The listing builds one solid part. Answer for the finished solid, in the listing's coordinates (mm). A direction names the side the tool comes from. Coordinates: 2 decimals unless noted, no trailing zeros. Write each loop counter-clockwise with the first axis right and the second up, starting at its lowest first coordinate (ties: lowest second). Pieces come first, ordered by that corner, then holes.
from build123d import *

# Parameters (mm, degrees)
BOSS_EXTRUDE1_DEPTH = 4.365625
SKETCH2_OUTSIDE_W   = 44.614
SKETCH2_OUTSIDE_H   = 45.964
SKETCH2_OUTSIDE_R   = 4.365625
CUT_EXTRUDE1_DEPTH  = 8.9705043
CUT_EXTRUDE1_DRAFT  = -60
SKETCH4_R           = 2.0828
CUT_EXTRUDE3_DEPTH  = 4.365625
SKETCH9_W           = 1.767564538
SKETCH9_H           = 1.190625


# Read off the part's stored shape, not the designer's step: Cut-Extrude4, Cut-Extrude5
with BuildPart() as part:
    # Sketch1 → Boss-Extrude1 (new body)
    with BuildSketch(Plane(origin=(0, 0, 0), x_dir=(1, 0, 0), z_dir=(0, 1, 0))):
        Polygon((0, 5.040989538), (-4.365625, 2.520494769), (-4.365625, -2.520494769), (0, -5.040989538), (4.365625, -2.520494769), (4.365625, 2.520494769), align=None)
    extrude(amount=BOSS_EXTRUDE1_DEPTH)


with BuildPart() as cut_extrude1_tool:
    # Sketch2 outside → Cut-Extrude1 (with draft: the straight prism first)
    with BuildSketch(Plane(origin=(0, 4.365625, 0), x_dir=(1, 0, 0), z_dir=(0, 1, 0))):
        Rectangle(SKETCH2_OUTSIDE_W, SKETCH2_OUTSIDE_H)
        Circle(SKETCH2_OUTSIDE_R, mode=Mode.SUBTRACT)
    extrude(amount=-CUT_EXTRUDE1_DEPTH)
    # Cut-Extrude1: the draft: its side faces are tilted about the plane it starts from
    cut_extrude1_sides = [cut_extrude1_tool.faces().sort_by_distance(p)[0] for p in [
        (0, -0.11962715, 22.982),
        (22.307, -0.11962715, 0),
        (0, -0.11962715, -22.982),
        (-22.307, -0.11962715, 0),
        (-4.365625, -0.11962715, 0),
    ]]
    draft(cut_extrude1_sides, Plane(origin=(0, 4.365625, 0), x_dir=(1, 0, 0), z_dir=(0, 1, 0)), CUT_EXTRUDE1_DRAFT)


with BuildPart() as part_1:
    add(part.part)

    # Cut-Extrude1: cut by cut_extrude1_tool
    add(cut_extrude1_tool.part, mode=Mode.SUBTRACT)

    # Sketch4 → Cut-Extrude3 (cut)
    with BuildSketch(Plane(origin=(0, 4.365625, 0), x_dir=(1, 0, 0), z_dir=(0, 1, 0))):
        with Locations(Location((0, 0, 0), (0, 0, 270))):
            Circle(SKETCH4_R)
    extrude(amount=-CUT_EXTRUDE3_DEPTH, mode=Mode.SUBTRACT)

    # Cut-Extrude4 outline → Cut-Extrude4 (revolve, cut)
    with BuildSketch(Plane.XY):
        Polygon((2.0828, 4.365625), (2.0828, 4.279699042), (2.168725958, 4.365625), align=None)
    revolve(axis=Axis((0, 0, 0), (0, 1, 0)), mode=Mode.SUBTRACT)

    # Cut-Extrude5 outline → Cut-Extrude5 (revolve, cut)
    with BuildSketch(Plane.XY):
        Polygon((2.168725958, 0), (2.0828, 0.085925958), (2.0828, 0), align=None)
    revolve(axis=Axis((0, 0, 0), (0, 1, 0)), mode=Mode.SUBTRACT)

    # Sketch9 → Cut-Revolve1 (revolve, cut)
    with BuildSketch(Plane(origin=(0, 0, 0), x_dir=(0, 0, -1), z_dir=(1, 0, 0)), mode=Mode.PRIVATE) as cut_revolve1_sk:
        with Locations((4.157207269, 0.5953125)):
            Rectangle(SKETCH9_W, SKETCH9_H)
    revolve(cut_revolve1_sk.sketch.rotate(Axis((0, 0, 0), (0, 1, 0)), 180), axis=Axis((0, 0, 0), (0, 1, 0)), mode=Mode.SUBTRACT)


solid = part_1.part
1. A tool of negligible diameter and unlimited length cuts with its end or side. For faces 1 (the flat face through (4.366, 3, 0)), 2 (the cylindrical face through (-2.904, 0.604, 1.51)), from which of +Z, -Z, +X, -X, +Y, -Y can it reach the whole face along a straight path? Write none if from no direction.
Results found:
face 1: +Z, -Z, +X, +Y, -Y
face 2: -Y
2. Find the intervals of material crossed by L1, parallel to X at y = 2.6, z = 0; L2, parallel to Y at x = -0.5, z = 3.75; L3, parallel to X at y = 0.5, z = -1.25, in increasing order.
Results found:
L1: x = -4.37 to -2.08, 2.08 to 4.37
L2: y = 1.19 to 4.37
L3: x = -3.03 to -1.67, 1.67 to 3.03
3. For a pull along X with two mould halves and no side action, classify faces 3 (the cylindrical face through (0.626, 2.212, 1.987)), 4 (the conical face through (3.915, 4.273, 2.273)), 5 (the conical face through (0.01, 4.27, -4.53)) as pulls with the +X half, pulls with the -X half, needs draft (parallel to the pull), parting line crosses it, or undercut.
Results found:
face 3: undercut
face 4: pulls with the +X half
face 5: parting line crosses it
4. Section A-A on y = 1.45 is taken. Give the vertices of the cut face in (x, z).
Results found:
outline: (-4.37, -2.52) - (0, -5.04) - (4.37, -2.52) - (4.37, 2.52) - (0, 5.04) - (-4.37, 2.52) - close; hole circle Ø4.17 at (0, 0)
5. Section B-B on y = 0.7 is taken. Give the vertices of the cut face in (x, z), then the cut area to 3 significant figures.
Results found:
outline: circle Ø6.55 at (0, 0); hole circle Ø4.17 at (0, 0)
area: 20.0 mm2
